Can you work these out from the model? Positions are in its coordinate system, mm. A direction names the side the tool comes from. Coordinates: 2 decimals unless noted, no trailing zeros. Loops run counter-clockwise (first coordinate to the right, second up) from the corner with the lowest first, then second, coordinate; pieces in that order, holes last.
```python
from build123d import *

# Parameters (mm, degrees)
BOSS_EXTRUDE1_DEPTH = 2
SKETCH2_R           = 7.5
BOSS_EXTRUDE2_DEPTH = 2
SKETCH3_R           = 2.5
BOSS_EXTRUDE3_DEPTH = 10
SKETCH4_R           = 0.75
BOSS_EXTRUDE4_DEPTH = 20
SKETCH5_R           = 1
BOSS_EXTRUDE5_DEPTH = 5
SKETCH6_W           = 14.887597411
SKETCH6_H           = 5
BOSS_EXTRUDE6_DEPTH = 61


with BuildPart() as part:
    # Sketch1 → Boss-Extrude1 (new body)
    with BuildSketch(Plane.XY):
        Polygon((7.397125851, -4.5036129), (7.598806105, 4.154292452), (0.201680255, 8.657905351), (-7.397125851, 4.5036129), (-7.598806105, -4.154292452), (-0.201680255, -8.657905351), align=None)
    extrude(amount=-BOSS_EXTRUDE1_DEPTH)

    # Sketch2 → Boss-Extrude2 (add)
    with BuildSketch(Plane.XY):
        with Locations(Location((0, 0, 0), (0, 0, 178.665573541))):
            Circle(SKETCH2_R)
    extrude(amount=BOSS_EXTRUDE2_DEPTH)

    # Sketch3 → Boss-Extrude3 (add)
    with BuildSketch(Plane.XY.offset(2)):
        Circle(SKETCH3_R)
    extrude(amount=BOSS_EXTRUDE3_DEPTH)

    # Sketch4 → Boss-Extrude4 (add)
    with BuildSketch(Plane.XY.offset(12)):
        Circle(SKETCH4_R)
    extrude(amount=BOSS_EXTRUDE4_DEPTH)

    # Sketch5 → Boss-Extrude5 (add)
    with BuildSketch(Plane.XY.offset(32)):
        Circle(SKETCH5_R)
    extrude(amount=BOSS_EXTRUDE5_DEPTH)

    # Sketch6 → Boss-Extrude6 (add)
    with BuildSketch(Plane(origin=(0, 0, -2), x_dir=(-1, 0, 0), z_dir=(0, 0, -1))):
        with Locations((0.034941521, -1.5)):
            Rectangle(SKETCH6_W, SKETCH6_H)
    extrude(amount=BOSS_EXTRUDE6_DEPTH)


solid = part.part
```
(1) I want a section at B-B on z = -56. Write out the boundary of the cut face in (x, y).
Check values:
outline: (-7.48, -4) - (7.41, -4) - (7.41, 1) - (-7.48, 1) - close
(2) I want a section at A-A on x = -6.5. Write out the boundary of the cut face in (y, z), then the cut area to 3 significant figures.
Check values:
outline: (-4.82, -2) - (-4, -2) - (-4, -63) - (1, -63) - (1, -2) - (4.99, -2) - (4.99, 0) - (3.74, 0) - (3.74, 2) - (-3.74, 2) - (-3.74, 0) - (-4.82, 0) - close
area: 340 mm2
(3) I'm going to push flat-ended pins straight in: pin 1 (5 mm diameter, centred on x = 6, z = 9, fed in from -Y); pin 2 (2 mm diameter, centred on x = -3, y = -2.5, fed in from +Z); pin 3 (1 mm diameter, centred on y = 2.5, z = 7.5, fed in from -X); pin 4 (4.5 mm diameter, centred on x = 1.5, z = -24.5, fed in from -Y). Where does each tip first touch, or does it pass through?
Check values:
pin 1: passes through
pin 2: stops at z = 2
pin 3: stops at x = -1.5
pin 4: stops at y = -4
(4) I want a section at C-C on x = 5. Write out the boundary of the cut face in (y, z), then the cut area to 3 significant figures.
Check values:
outline: (-5.81, -2) - (-4, -2) - (-4, -63) - (1, -63) - (1, -2) - (5.74, -2) - (5.74, 0) - (5.59, 0) - (5.59, 2) - (-5.59, 2) - (-5.59, 0) - (-5.81, 0) - close
area: 350 mm2
(5) Which directions (+Z, -Z, +X, -X, +Y, -Y) give clear straight access to the entire face, cutting with the end or side of a thin tool? Please do faces 1 (the flat face through (7.409, -2, -32)), 2 (the flat face through (0, 1, -32)), 3 (the flat face through (-7, -4, 0)).
Check values:
face 1: -Z, +X, +Y, -Y
face 2: -Z, +X, -X, +Y
face 3: +Z, -X, -Y
(6) If I drill on probe 1 along Y at (x, z) = (3, -15); probe 2 along Z at (x, y) = (-5.5, -2.5); probe 3 along Z at (x, y) = (-5.5, 3), over which ranges is the centre line in solid material (lowest first)?
Check values:
probe 1: y = -4 to 1
probe 2: z = -63 to 2
probe 3: z = -2 to 2
